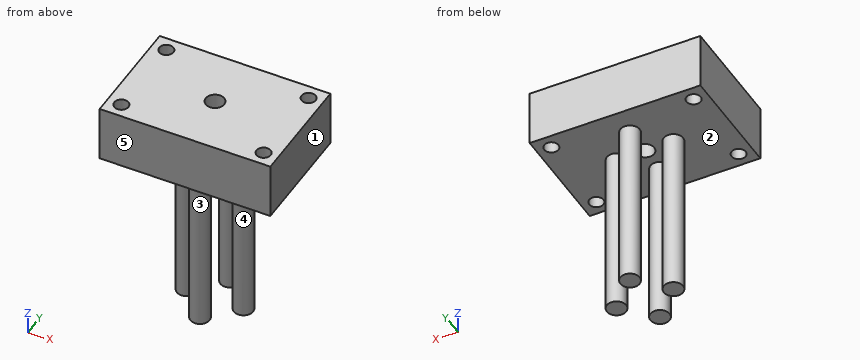
from build123d import *

# Parameters (mm, degrees)
SKETCH1_W           = 76.2
SKETCH1_H           = 50.8
SKETCH1_R           = 4.31365531
BOSS_EXTRUDE2_DEPTH = 25.4
SKETCH6_R           = 4.1275
SKETCH6_R_2         = 3.175
CUT_EXTRUDE3_DEPTH  = 25.4
BOSS_EXTRUDE3_START = -101.6
SKETCH7_R           = 4.31365531
BOSS_EXTRUDE3_DEPTH = 101.6
BOSS_EXTRUDE5_START = -101.6
SKETCH9_R           = 4.31365531
BOSS_EXTRUDE5_DEPTH = 101.6
SKETCH11_R          = 4.316155828
BOSS_EXTRUDE6_DEPTH = 101.6
BOSS_EXTRUDE7_START = -101.6
SKETCH14_R          = 4.31365531
BOSS_EXTRUDE7_DEPTH = 101.6


with BuildPart() as part:
    # Sketch1 → Boss-Extrude2 (new body)
    with BuildSketch(Plane.XY):
        with Locations((38.1, 25.4)):
            Rectangle(SKETCH1_W, SKETCH1_H)
        with Locations((38.1, 38.1)):
            Circle(SKETCH1_R, mode=Mode.SUBTRACT)
        with Locations((50.8, 25.4)):
            Circle(SKETCH1_R, mode=Mode.SUBTRACT)
        with Locations((38.1, 12.7)):
            Circle(SKETCH1_R, mode=Mode.SUBTRACT)
        with Locations((25.4, 25.4)):
            Circle(SKETCH1_R, mode=Mode.SUBTRACT)
    extrude(amount=BOSS_EXTRUDE2_DEPTH)

    # Sketch6 → Cut-Extrude3 (cut)
    with BuildSketch(Plane.XY.offset(25.4)):
        with Locations((38.1, 25.4)):
            Circle(SKETCH6_R)
        with Locations((6.35, 44.45)):
            Circle(SKETCH6_R_2)
        with Locations((69.85, 44.45)):
            Circle(SKETCH6_R_2)
        with Locations((6.35, 6.35)):
            Circle(SKETCH6_R_2)
        with Locations((69.85, 6.35)):
            Circle(SKETCH6_R_2)
    extrude(amount=-CUT_EXTRUDE3_DEPTH, mode=Mode.SUBTRACT)

    # Sketch7 → Boss-Extrude3 (add)
    with BuildSketch(Plane.XY.offset(25.4).offset(BOSS_EXTRUDE3_START)):
        with Locations((25.4, 25.4)):
            Circle(SKETCH7_R)
    extrude(amount=BOSS_EXTRUDE3_DEPTH)

    # Sketch9 → Boss-Extrude5 (add)
    with BuildSketch(Plane.XY.offset(25.4).offset(BOSS_EXTRUDE5_START)):
        with Locations((50.8, 25.4)):
            Circle(SKETCH9_R)
    extrude(amount=BOSS_EXTRUDE5_DEPTH)

    # Sketch11 → Boss-Extrude6 (add)
    with BuildSketch(Plane.XY.offset(25.4)):
        with Locations((38.097842062, 38.101263286)):
            Circle(SKETCH11_R)
    extrude(amount=-BOSS_EXTRUDE6_DEPTH)

    # Sketch14 → Boss-Extrude7 (add)
    with BuildSketch(Plane.XY.offset(25.4).offset(BOSS_EXTRUDE7_START)):
        with Locations((38.1, 12.7)):
            Circle(SKETCH14_R)
    extrude(amount=BOSS_EXTRUDE7_DEPTH)


solid = part.part
CAD build for the part. Positions are in the model's coordinates, mm. Face numbers are marked on the shaded views. A direction names the side the tool comes from. Round coordinates to 2 decimals unless told otherwise and drop trailing zeros. Order: outer loops, then holes, each group sorted by start corner. A loop starts at its lowest first (then second) coordinate and runs counter-clockwise, first axis right, second up. Notation, with made-up numbers: M 20,73.5 L 72,73.5 A29 cw 72,111.5 Z; hole C 37.25,-4 d1. An arc over 180 degrees is marked long. Use one line per item in the form item = value.
Q1. Saw through at D-D on y = 12.7. Give the cut face in (x, z), then the cut area to 3 significant figures.
Recorded:
outline = M 0,0 L 33.79,0 L 33.79,-76.2 L 42.41,-76.2 L 42.41,0 L 76.2,0 L 76.2,25.4 L 0,25.4 Z
area = 2,590 mm^2
Q2. Saw through at A-A on x = 69.85. Give the cut face in (y, z) (3 decimals).
Recorded:
outline = M 0,0 L 3.175,0 L 3.175,25.4 L 0,25.4 Z; M 9.525,0 L 41.275,0 L 41.275,25.4 L 9.525,25.4 Z; M 47.625,0 L 50.8,0 L 50.8,25.4 L 47.625,25.4 Z
Q3. Saw through at B-B on y = 44.45. Give the cut face in (x, z) (3 decimals), then the cut area to 3 significant figures.
Recorded:
outline = M 0,0 L 3.175,0 L 3.175,25.4 L 0,25.4 Z; M 9.525,0 L 66.675,0 L 66.675,25.4 L 9.525,25.4 Z; M 73.025,0 L 76.2,0 L 76.2,25.4 L 73.025,25.4 Z
area = 1,610 mm^2
Q4. Flat gauge pins, fed straight in: P1, Ø8, axis at x = 20.5, z = -36, coming from the +Y side; P2, Ø5, axis at x = 36, z = -24.5, coming from the +Y side; P3, Ø10, axis at y = 41.5, z = -11, coming from the -X side. Where does each tip first touch, or does it go through?
Recorded:
P1 = 29.62
P2 = 42.42
P3 = 33.78
Q5. Two-plate mould, pull along X, no slides. Class the marked faces 3, 4 and 5: +X half, -X half, draft (parallel to the pull), parting line (faces both ways), or undercut.
Recorded:
face_3 = parting line
face_4 = undercut
face_5 = draft
Q6. Which spindle directions (+Z, -Z, +X, -X, +Y, -Y) get a long thin tool onto all of the face, cutting with end or side? Do the marked faces 1 and 2. Say none if no direction does.
Recorded:
face_1 = +Z, -Z, +X, +Y, -Y
face_2 = -Z
Q7. Probe L1, parallel to Y at x = 6.35, z = 12 (3 decimals); L2, parallel to X at y = 6, z = 10; L3, parallel to Y at x = 72, z = 11. List the from-to ranges inside material, lowest first.
Recorded:
L1 = 0 to 3.175, 9.525 to 41.275, 47.625 to 50.8
L2 = 0 to 3.19, 9.51 to 66.69, 73.01 to 76.2
L3 = 0 to 4.01, 8.69 to 42.11, 46.79 to 50.8
Q8. Saw through at C-C on z = 5. State how many separate pieces and enclosed holes the cut face has, then the cut area to 3 significant figures.
Recorded:
separate_pieces = 1
enclosed_holes = 5
area = 3,690 mm^2
